Can you work these out from the model? Positions are in its coordinate system, mm. A direction names the side the tool comes from. Round coordinates to 2 decimals unless told otherwise and drop trailing zeros. Loops run counter-clockwise (first coordinate to the right, second up) from the corner with the lowest first, then second, coordinate; pieces in that order, holes last. Notation, with made-up numbers: (-5.5, 68) -> (46.5, 68) arc R28 ccw to (46.5, 104) -> close; hole circle Ø11 at (51.5, -29). An arc over 180 degrees is marked (long way). Use a Markdown table: item, result.
Autodesk Inventor part; units mm, degrees
ref_plane "YZ Plane" through (0, 0, 0) normal (1, 0, 0) x (0, 1, 0)
ref_plane "XZ Plane" through (0, 0, 0) normal (0, 1, 0) x (-1, 0, 0)
ref_plane "XY Plane" through (0, 0, 0) normal (0, 0, 1) x (1, 0, 0)
sketch "Sketch1" plane through (0, 0, 0) normal (0, 0, 1) x (1, 0, 0)
  arc A0 (22.225, 45.6803) -> (-22.225, 45.6803) centre (0, 0) ccw
  line L0 (-22.225, 45.6803) -> (-22.225, 73.66)
  line L1 (-22.225, 73.66) -> (22.225, 73.66)
  line L2 (22.225, 73.66) -> (22.225, 45.6803)
  line L3 (0, 73.66) -> (0, 50.8) construction
  line L4 (-22.225, 73.66) -> (-19.685, 73.66)
  line L5 (-19.685, 73.66) -> (-19.685, 80.01)
  line L6 (-19.685, 80.01) -> (-22.225, 80.01)
  line L7 (-22.225, 80.01) -> (-22.225, 73.66)
  line L8 (22.225, 73.66) -> (19.685, 73.66)
  line L9 (19.685, 73.66) -> (19.685, 80.01)
  line L10 (19.685, 80.01) -> (22.225, 80.01)
  line L11 (22.225, 80.01) -> (22.225, 73.66)
  dimension "d0" = 101.6
  dimension "d1" = 44.45
  dimension "d2" = 22.86
  dimension "d3" = 2.54
  dimension "d4" = 6.35
  dimension "d5" = 2.54
  dimension "d6" = 6.35
extrude "Extrusion1" add sketch "Sketch1" along normal blind 38.1
sketch "Sketch2" plane through (0, 0, 38.1) normal (0, 0, 1) x (1, 0, 0)
  line L0 (-19.685, 80.01) -> (-22.225, 80.01)
  line L1 (-22.225, 80.01) -> (-22.225, 45.6803)
  line L2 (22.225, 80.01) -> (19.685, 80.01)
  line L3 (22.225, 45.6803) -> (22.225, 80.01)
  line L4 (-19.685, 80.01) -> (-23.495, 85.09)
  line L5 (-23.495, 85.09) -> (-26.67, 85.09)
  line L6 (-26.67, 85.09) -> (-22.225, 79.1633)
  line L7 (19.685, 80.01) -> (23.495, 85.09)
  line L8 (23.495, 85.09) -> (26.67, 85.09)
  line L9 (26.67, 85.09) -> (22.225, 79.1633)
  line L10 (-23.495, 85.09) -> (23.495, 85.09) construction
  line L11 (19.685, 73.66) -> (-19.685, 73.66) construction
  point P0 (0, 0)
  point P1 (0, 85.09)
  point P2 (0, 73.66)
  dimension "d9" = 2.54
  dimension "d10" = 2.54
  dimension "d11" = 5.08
  dimension "d12" = 46.99
extrude "Extrusion2" add sketch "Sketch2" against normal up to surface (38.1 mm away)
sketch "Sketch3" plane through (0, 0, 0) normal (0, 1, 0) x (-1, 0, 0)
  line L0 (0, 0) -> (26.67, 25.4)
  line L1 (26.67, 38.1) -> (26.67, 0)
  line L2 (26.67, 0) -> (23.495, 0)
  line L3 (26.67, 0) -> (26.67, 25.4)
  line L4 (26.67, 0) -> (0, 0)
  line L5 (0, 0) -> (-26.67, 25.4)
  line L6 (-26.67, 38.1) -> (-26.67, 0)
  line L7 (-26.67, 25.4) -> (-26.67, 0)
  line L8 (-26.67, 0) -> (0, 0)
  dimension "d15" = 25.4
extrude "Extrusion3" cut sketch "Sketch3" along normal through all
fillet "Fillet1" radius 3.175 3 edges at (0, 62.23, 0) (22.225, 62.4218, 21.1667) (-22.225, 62.4218, 21.1667)
fillet "Fillet2" radius 0.635 2 edges at (26.67, 85.09, 31.75) (-26.67, 85.09, 31.75)
equation "\"d10\" = d9"
properties part number "aftMount" material "ABS Plastic"
1. If we mould it in two halves opening along X, with no side actions, what happens to faces 1 (the flat face through (11.3, 61.02, 10.76)), 2 (the flat face through (0, 61, 38.1)), 3 (the cylindrical face through (-0.3, 50.8, 23.5)), 4 (the flat face through (19.685, 77, 28))? For each: +X half, -X half, draft (parallel to the pull), parting line (faces both ways), or undercut.
Answer sheet:
| item | result |
|---|---|
| face 1 | +X half |
| face 2 | draft |
| face 3 | undercut |
| face 4 | undercut |
2. I want a section at B-B (y = 67). Please give me the cut outline in (x, z) (3 decimals), plus the area to 3 significant figures.
Answer sheet:
| item | result |
|---|---|
| outline | (-22.225, 22.527) arc R3.175 ccw to (-21.24, 20.228) -> (-2.19, 2.085) arc R3.175 ccw to (2.19, 2.085) -> (21.24, 20.228) arc R3.175 ccw to (22.225, 22.527) -> (22.225, 38.1) -> (-22.225, 38.1) -> close |
| area | 1,220 mm² |
3. Which directions (+Z, -Z, +X, -X, +Y, -Y) give clear straight access to the entire face, cutting with the end or side of a thin tool? Please do faces 5 (the cylindrical face through (21.975, 62.656, 21.293)), 6 (the cylindrical face through (-21.96, 62.66, 21.26)), 7 (the flat face through (0, 73.66, 23)).
Answer sheet:
| item | result |
|---|---|
| face 5 | -Z, +X, -Y |
| face 6 | -Z, -X, -Y |
| face 7 | +Z, -Z, +Y |
4. I want a section at A-A (z = 30.5). Please give me the cut outline in (x, y) (3 decimals), plus the area to 3 significant figures.
Answer sheet:
| item | result |
|---|---|
| outline | (-25.908, 84.074) -> (-22.225, 79.163) -> (-22.225, 45.68) arc R50.8 cw to (22.225, 45.68) -> (22.225, 79.163) -> (25.908, 84.074) arc R0.635 ccw to (25.4, 85.09) -> (23.495, 85.09) -> (19.685, 80.01) -> (19.685, 73.66) -> (-19.685, 73.66) -> (-19.685, 80.01) -> (-23.495, 85.09) -> (-25.4, 85.09) arc R0.635 ccw to start |
| area | 1,150 mm² |
5. I need wall thicknesses on line 1 (X direction, y = 71, z = 32) (3 decimals); line 2 (X direction, y = 76, z = 19) (3 decimals); line 3 (X direction, y = 75.5, z = 21) (3 decimals). Which ranges of each line are inside material? Lowest first, please.
Answer sheet:
| item | result |
|---|---|
| line 1 | x = -22.225 to 22.225 |
| line 2 | x = -19.95 to -19.685, 19.685 to 19.95 |
| line 3 | x = -21.833 to -19.685, 19.685 to 21.833 |
6. I want a section at C-C (x = 0). Please give me the cut outline in (y, z).
Answer sheet:
| item | result |
|---|---|
| outline | (50.8, 1.21) -> (73.66, 1.21) -> (73.66, 38.1) -> (50.8, 38.1) -> close |
7. Will these pins go through, and if not, where does the flat tip stop? pin 1 Ø12.5 at (y, z) = (54.5, 33.5) entering from -X (3 decimals); pin 2 Ø1 at (y, z) = (79.5, 18.5) entering from -X; pin 3 Ø3 at (x, z) = (18, 20.5) entering from -Y; pin 4 Ø1 at (y, z) = (75.5, 16) entering from -X.
Answer sheet:
| item | result |
|---|---|
| pin 1 | stops at x = -22.225 |
| pin 2 | stops at x = -19.95 |
| pin 3 | stops at y = 46.91 |
| pin 4 | passes through |
8. I want a section at D-D (z = 16). Please give me the cut outline in (x, y), plus the area to 3 significant figures.
Answer sheet:
| item | result |
|---|---|
| outline | (-16.8, 47.94) arc R50.8 cw to (16.8, 47.94) -> (16.8, 73.66) -> (-16.8, 73.66) -> close |
| area | 800 mm² |
